Build history of the part. All positions in model axes, mm. Give positions to 0.01 mm unless a question says otherwise; leave off trailing zeros. Loops run counter-clockwise (first coordinate to the right, second up) from the corner with the lowest first, then second, coordinate; pieces in that order, holes last. Notation, with made-up numbers: M 20,75 L 34,75 A18 ccw 34,102 Z; hole C -5,-24 d10. An arc over 180 degrees is marked long. Answer as a JSON object with one key per item and string values. Group by question number.
1. Drill centre lines: line 1 along Z through (x, y) = (0.1, -183); line 2 along Z through (x, y) = (0.7, -197.45); line 3 along Y through (x, z) = (0.7, 179.5). Where is each one in solid material? Low to high. Write a range as [from, to].
2. Drop flat-ended pins along their axis: pin 1 Ø3 at (y, z) = (-161, 163.5) entering from -X; pin 2 Ø2.5 at (y, z) = (-87, 19.18) entering from +X; pin 3 Ø0.9 at (x, z) = (1.5, 137) entering from +Y. Give the stop position or say it passes through.
3. Slice it at B-B (x = 2.35). Give the number of separate pieces and of enclosed holes in the cut face, then the cut area to 3 significant figures.
4. Slice it at A-A (y = -40.5). List the corners of the cut face in (x, z), then the cut area to 3 significant figures.
Solid Edge part; units mm, degrees
sketch "Sketch1" plane through (0, 0, 0) normal (-1, 0, 0) x (0, -1, 0)
  line L0 (0, 0) -> (207.45, 0)
  line L1 (207.45, 0) -> (207.45, 214.47)
  line L2 (207.45, 214.47) -> (0, 214.47)
  line L3 (0, 214.47) -> (0, 0)
extrude "Protrusion1" add sketch "Sketch1" against normal blind 3
sketch "Sketch2" plane through (0, -103.725, 107.235) normal (-1, 0, 0) x (0, 1, 0)
  line L0 (-83.975, -28.235) -> (114.48, -28.235)
  line L1 (114.48, -28.235) -> (114.48, -31.235)
  line L2 (-83.975, -31.235) -> (114.48, -31.235)
  line L3 (-83.975, -28.235) -> (-83.975, -31.235)
  line L4 (-83.975, 11.765) -> (114.48, 11.765)
  line L5 (114.48, 11.765) -> (114.48, 14.765)
  line L6 (-83.975, 14.765) -> (114.48, 14.765)
  line L7 (-83.975, 11.765) -> (-83.975, 14.765)
  line L8 (-83.975, 57.765) -> (114.48, 57.765)
  line L9 (114.48, 57.765) -> (114.48, 54.765)
  line L10 (-83.975, 54.765) -> (114.48, 54.765)
  line L11 (-83.975, 57.765) -> (-83.975, 54.765)
  line L12 (-83.975, -74.235) -> (114.48, -74.235)
  line L13 (114.48, -74.235) -> (114.48, -71.235)
  line L14 (-83.975, -71.235) -> (114.48, -71.235)
  line L15 (-83.975, -74.235) -> (-83.975, -71.235)
  line L16 (-83.975, -104.235) -> (114.48, -104.235)
  line L17 (114.48, -104.235) -> (114.48, -107.235)
  line L18 (-83.975, -107.235) -> (114.48, -107.235)
  line L19 (-83.975, -104.235) -> (-83.975, -107.235)
  dimension "D1" = 114.48
  dimension "D2" = 83.975
  dimension "D3" = 114.48
  dimension "D4" = 83.975
extrude "Cutout1" cut sketch "Sketch2" against normal blind 10
sketch "Sketch3" plane through (0, -103.725, 107.235) normal (-1, 0, 0) x (0, 1, 0)
  line L0 (-118.847, 97.765) -> (179.5114, 97.765)
  line L1 (191.0928, 110.2989) -> (179.5114, 97.765)
  line L2 (-118.847, 116.9168) -> (191.0928, 110.2989)
  line L3 (-118.847, 97.765) -> (-118.847, 116.9168)
extrude "Cutout2" cut sketch "Sketch3" against normal blind 37
sketch "Sketch4" plane through (0, -103.725, 111.97) normal (-1, 0, 0) x (0, 1, 0)
  line L0 (-103.725, 102.5) -> (-103.725, -102.5)
  line L1 (-103.725, -102.5) -> (83.725, -102.5)
  line L2 (83.725, -102.5) -> (83.725, -99.5)
  line L3 (83.725, -99.5) -> (103.725, -99.5)
  line L4 (103.725, -99.5) -> (103.725, -69.5)
  line L5 (83.725, -69.5) -> (103.725, -69.5)
  line L6 (83.725, -66.5) -> (83.725, -69.5)
  line L7 (83.725, -66.5) -> (103.725, -66.5)
  line L8 (103.725, -66.5) -> (103.725, -26.5)
  line L9 (83.725, -26.5) -> (103.725, -26.5)
  line L10 (83.725, -23.5) -> (83.725, -26.5)
  line L11 (83.725, -23.5) -> (103.725, -23.5)
  line L12 (103.725, -23.5) -> (103.725, 16.5)
  line L13 (83.725, 16.5) -> (103.725, 16.5)
  line L14 (83.725, 19.5) -> (83.725, 16.5)
  line L15 (83.725, 19.5) -> (103.725, 19.5)
  line L16 (103.725, 19.5) -> (103.725, 59.5)
  line L17 (83.725, 59.5) -> (103.725, 59.5)
  line L18 (83.725, 62.5) -> (83.725, 59.5)
  line L19 (83.725, 62.5) -> (103.725, 62.5)
  line L20 (103.725, 62.5) -> (103.725, 102.5)
  line L21 (32.3413, 102.5) -> (103.725, 102.5)
  line L22 (-103.725, 102.5) -> (32.3413, 102.5)
  dimension "D1" = 103.725
extrude "Protrusion2" add sketch "Sketch4" along normal blind 3
sketch "Sketch5" plane through (0, -113.725, 214.47) normal (0, 0, 1) x (0, 1, 0)
  line L0 (-93.725, -3) -> (113.725, -3)
  line L1 (113.725, -3) -> (113.725, 3)
  line L2 (113.725, 3) -> (-93.725, 3)
  line L3 (-93.725, 3) -> (-93.725, -3)
extrude "Protrusion3" add sketch "Sketch5" along normal blind 15
sketch "Sketch6" plane through (-3, -103.725, 111.8236) normal (-1, 0, 0) x (0, 1, 0)
  circle A0 centre (93.725, 92.6464) radius 2
  circle A1 centre (16.725, 92.6464) radius 2
  circle A2 centre (-16.725, 92.6464) radius 2
  circle A3 centre (-93.725, -107.9393) radius 2
  circle A4 centre (93.725, -107.9393) radius 2
  circle A5 centre (16.725, -107.9393) radius 2
  circle A6 centre (-16.725, -107.9393) radius 2
  circle A7 centre (-93.725, 92.6464) radius 2
  dimension "D1" = 93.725
  dimension "D2" = 93.725
extrude "Cutout3" cut sketch "Sketch6" against normal blind 10
sketch "Sketch7" plane through (0, -103.725, 229.47) normal (0, 0, 1) x (0, 1, 0)
  line L0 (-110.3839, 0) -> (-110.3839, 8.5479)
  line L1 (-110.3839, 8.5479) -> (109.9811, 8.5479)
  line L2 (109.9811, 8.5479) -> (111.4132, 0)
  line L3 (111.4132, 0) -> (-110.3839, 0)
extrude "ExtrudedCutout_41" cut sketch "Sketch7" against normal blind 407
sketch "Sketch8" plane through (3, -103.725, 119.47) normal (1, 0, 0) x (0, 1, 0)
  line L0 (96.275, 123.6289) -> (96.275, -147.9139)
  line L1 (117.9514, -132.6396) -> (96.275, -147.9139)
  line L2 (117.9514, 110.6175) -> (117.9514, -132.6396)
  line L3 (96.275, 123.6289) -> (117.9514, 110.6175)
extrude "ExtrudedCutout_42" cut sketch "Sketch8" against normal blind 43
Established:
{
 "1": {"line 1": "z = [9.47, 49.47], [52.47, 92.47], [95.47, 135.47], [138.47, 178.47], [181.47, 211.47], [214.47, 229.47]", "line 2": "z = [9.47, 17.18], [21.18, 217.76], [221.76, 229.47]", "line 3": "y = [-207.45, -187.7]"},
 "2": {"pin 1": "stops at x = 0", "pin 2": "passes through", "pin 3": "stops at y = -187.7"},
 "3": {"separate pieces": "1", "enclosed holes": "8", "area": "41,200 mm^2"},
 "4": {"outline": "M 0,9.47 L 3,9.47 L 3,49.47 L 0,49.47 Z; M 0,52.47 L 3,52.47 L 3,92.47 L 0,92.47 Z; M 0,95.47 L 3,95.47 L 3,135.47 L 0,135.47 Z; M 0,138.47 L 3,138.47 L 3,178.47 L 0,178.47 Z; M 0,181.47 L 3,181.47 L 3,211.47 L 0,211.47 Z; M 0,214.47 L 3,214.47 L 3,229.47 L 0,229.47 Z", "area": "615 mm^2"}
}
